The model under review builds one solid part; all positions refer to its coordinate system, in mm. A direction names the side the tool comes from. Round coordinates to 2 decimals unless told otherwise and drop trailing zeros. Order: outer loops, then holes, each group sorted by start corner. A loop starts at its lowest first (then second) coordinate and runs counter-clockwise, first axis right, second up. Notation, with made-up numbers: M 41,0.25 L 69,0.25 A15 cw 69,27.25 Z; hole C 70,86 d5. An arc over 180 degrees is marked long. Use a Markdown table: item, result. Add a question column.
1. To check wall thickness, follow probe 1 along Y at (x, z) = (19, -5) (3 decimals); probe 2 along Y at (x, z) = (18, -15) (3 decimals); probe 3 along X at (y, z) = (-56.5, -2) (3 decimals). State the ranges of each line that lie inside material, in increasing order.
2. Consider section D-D on x = 33. State the section outline as (y, z) points (3 decimals).
3. Consider section A-A on x = 17. State the section outline as (y, z) points (3 decimals).
4. Consider section B-B on y = -86.5. State the section outline as (x, z) points (3 decimals), then the cut area to 3 significant figures.
5. For faces 5 (the flat face through (4.6, -67.3, 0)), 6 (the cylindrical face through (7.384, -75.99, -4.696)), list the 3-axis set-ups (+Z, -Z, +X, -X, +Y, -Y) from which the entire face can be reached by the end or side of a thin tool; tool diameter is ignored.
6. The part is to be moulded in two halves that separate along X. For faces 1 (the flat face through (33.32, -67.31, -1.57)), 2 (the flat face through (1.61, -67.307, -1.565)), 3 (the flat face through (14, -71, -9.525)), 4 (the flat face through (13, -67, -19.05)), say which applies: +X half, -X half, draft (parallel to the pull), parting line (faces both ways), or undercut.
from build123d import *

# Parameters (mm, degrees)
F0_W     = 34.925
F0_H     = 19.05
F1_DEPTH = 136.525
F2_SIZE  = 3.175
F3_R     = 12.7
F4_DEPTH = 9.525
F5_R     = 3.96875
F6_DEPTH = 254


with BuildPart() as f1:
    # F0 (on Front) → F1 (new body)
    with BuildSketch(Plane.XZ):
        with Locations((17.4625, -9.525)):
            Rectangle(F0_W, F0_H)
    extrude(amount=F1_DEPTH)

    # F2
    f2_edges = [f1.edges().sort_by_distance(p)[0] for p in [
        (34.925, -68.2625, 0),
        (0, -68.2625, 0),
    ]]
    chamfer(f2_edges, length=F2_SIZE)

    # F3 (on face) → F4 (cut)
    with BuildSketch(Plane.XY):
        with Locations((17.4625, -68.2625)):
            Circle(F3_R)
    extrude(amount=-F4_DEPTH, mode=Mode.SUBTRACT)

    # F5 (on face) → F6 (cut)
    with BuildSketch(Plane.XY.offset(-9.525)):
        with Locations((17.4625, -68.2625)):
            Circle(F5_R)
    extrude(amount=-F6_DEPTH, mode=Mode.SUBTRACT)


solid = f1.part
Answer block:
| question | item | result |
|---|---|---|
| 1 | probe 1 | -136.525 to -80.869, -55.656 to 0 |
| 1 | probe 2 | -136.525 to -72.195, -64.33 to 0 |
| 1 | probe 3 | 1.175 to 12.674, 22.251 to 33.75 |
| 2 | outline | M -136.525,-19.05 L 0,-19.05 L 0,-1.25 L -136.525,-1.25 Z |
| 3 | outline | M -136.525,-19.05 L -72.204,-19.05 L -72.204,-9.525 L -80.954,-9.525 L -80.954,0 L -136.525,0 Z; M -64.321,-19.05 L 0,-19.05 L 0,0 L -55.571,0 L -55.571,-9.525 L -64.321,-9.525 Z |
| 4 | outline | M 0,-19.05 L 34.925,-19.05 L 34.925,-3.175 L 31.75,0 L 3.175,0 L 0,-3.175 Z |
| 4 | area | 655 mm^2 |
| 5 | face 5 | +Z, +X, -X, +Y, -Y |
| 5 | face 6 | +Z |
| 6 | face 1 | +X half |
| 6 | face 2 | -X half |
| 6 | face 3 | undercut |
| 6 | face 4 | draft |
